from build123d import *

# Parameters (mm, degrees)
SKETCH1_W           = 53.32
SKETCH1_H           = 53.32
BOSS_EXTRUDE1_DEPTH = 5.08
SKETCH2_W           = 5.08
SKETCH2_H           = 5.08
CUT_EXTRUDE1_DEPTH  = 5.08
CUT_EXTRUDE2_DEPTH  = 5.08


with BuildPart() as part:
    # Sketch1 → Boss-Extrude1 (new body)
    with BuildSketch(Plane(origin=(0, 0, 0), x_dir=(1, 0, 0), z_dir=(0, 1, 0))):
        with Locations((4.159716312, -8.981205674)):
            Rectangle(SKETCH1_W, SKETCH1_H)
    extrude(amount=BOSS_EXTRUDE1_DEPTH)

    # Sketch2 → Cut-Extrude1 (cut)
    with BuildSketch(Plane(origin=(0, 5.08, 0), x_dir=(1, 0, 0), z_dir=(0, 1, 0))):
        with Locations((-13.620283688, -33.101205674)):
            Rectangle(SKETCH2_W, SKETCH2_H)
        with Locations((11.779716312, -33.101205674)):
            Rectangle(SKETCH2_W, SKETCH2_H)
        with Locations((21.939716312, -33.101205674)):
            Rectangle(SKETCH2_W, SKETCH2_H)
        with Locations((-3.460283688, -33.101205674)):
            Rectangle(SKETCH2_W, SKETCH2_H)
        with Locations((-19.960283688, 8.798794326)):
            Rectangle(SKETCH2_W, SKETCH2_H)
        with Locations((-19.960283688, -16.601205674)):
            Rectangle(SKETCH2_W, SKETCH2_H)
        with Locations((-19.960283688, -26.761205674)):
            Rectangle(SKETCH2_W, SKETCH2_H)
        with Locations((-19.960283688, -1.361205674)):
            Rectangle(SKETCH2_W, SKETCH2_H)
        with Locations((21.939716312, 15.138794326)):
            Rectangle(SKETCH2_W, SKETCH2_H)
        with Locations((-3.460283688, 15.138794326)):
            Rectangle(SKETCH2_W, SKETCH2_H)
        with Locations((-13.620283688, 15.138794326)):
            Rectangle(SKETCH2_W, SKETCH2_H)
        with Locations((11.779716312, 15.138794326)):
            Rectangle(SKETCH2_W, SKETCH2_H)
        with Locations((28.279716312, -26.761205674)):
            Rectangle(SKETCH2_W, SKETCH2_H)
        with Locations((28.279716312, -1.361205674)):
            Rectangle(SKETCH2_W, SKETCH2_H)
        with Locations((28.279716312, 8.798794326)):
            Rectangle(SKETCH2_W, SKETCH2_H)
        with Locations((28.279716312, -16.601205674)):
            Rectangle(SKETCH2_W, SKETCH2_H)
    extrude(amount=-CUT_EXTRUDE1_DEPTH, mode=Mode.SUBTRACT)

    # Sketch3 → Cut-Extrude2 (cut)
    with BuildSketch(Plane(origin=(0, 5.08, 0), x_dir=(1, 0, 0), z_dir=(0, 1, 0))):
        Polygon((4.159716312, -1.361205674), (6.699716312, -1.361205674), (6.699716312, -6.441205674), (11.779716312, -6.441205674), (11.779716312, -8.981205674), (11.779716312, -11.521205674), (6.699716312, -11.521205674), (6.699716312, -16.601205674), (4.159716312, -16.601205674), (1.619716312, -16.601205674), (1.619716312, -11.521205674), (-3.460283688, -11.521205674), (-3.460283688, -8.981205674), (-3.460283688, -6.441205674), (1.619716312, -6.441205674), (1.619716312, -1.361205674), align=None)
    extrude(amount=-CUT_EXTRUDE2_DEPTH, mode=Mode.SUBTRACT)


solid = part.part
Source: CAD feature listing. Evaluate the final solid. Frame: model axes, mm. A direction names the side the tool comes from. Give positions to 0.01 mm unless a question says otherwise; leave off trailing zeros. Write each loop counter-clockwise with the first axis right and the second up, starting at its lowest first coordinate (ties: lowest second). Pieces come first, ordered by that corner, then holes. Notation, with made-up numbers: (-24, 58.5) - (4, 58.5) arc R31 cw to (4, 97.5) - close; hole circle Ø4 at (70, 37.5). An arc over 180 degrees is marked (long way). Write item = value, one per line. Start each with the question number.
Q1. Material intervals for probe 1 along Z at (x, y) = (-18.5, 4.35); probe 2 along X at (y, z) = (0.3, -14); probe 3 along Z at (x, y) = (11, 4.65), sorted ascending.
Q2. Reachability of faces 4 (the flat face through (-14, 3, -12.599)), 5 (the flat face through (-6, 3, 33)), 6 (the flat face through (-20, 3, 3.901)), 7 (the flat face through (28, 3, -6.259)), 8 (the flat face through (9, 3, 6.441)) from +Z, -Z, +X, -X, +Y, -Y: full face, straight path, thin tool, end or side. Return the list, or none.
Q3. Pin query (flat end, axial travel): pin 1 Ø2.5 at (y, z) = (2.5, 26) entering from -X. Return the tip coordinate at first contact, or that it passes through.
Q4. Cut plane C-C, the plane x = 27. Return loops of the section in (y, z), then the cut area to 3 significant figures.
Q5. Cut plane A-A, the plane z = 5. Return loops of the section in (x, y), then the cut area to 3 significant figures.
Q6. Draft query along X for faces 1 (the flat face through (12, 3, -12.599)), 2 (the flat face through (30.82, 3, 33)), 3 (the flat face through (28, 3, -1.179)). Return one class per face: +X half, -X half, draft (parallel to the pull), parting line (faces both ways), or undercut.
Q7. Cut plane B-B, the plane x = 7.5. Return loops of the section in (y, z), then the cut area to 3 significant figures.
Computed values:
q1.probe_1 = -17.68 to -11.34, -6.26 to -1.18, 3.9 to 14.06, 19.14 to 24.22, 29.3 to 35.64
q1.probe_2 = -22.5 to -16.16, -11.08 to -6, -0.92 to 9.24, 14.32 to 19.4, 24.48 to 30.82
q1.probe_3 = -12.6 to 6.44, 11.52 to 30.56
q2.face_4 = -Z, +Y, -Y
q2.face_5 = +Z, +Y, -Y
q2.face_6 = -X, +Y, -Y
q2.face_7 = +X, +Y, -Y
q2.face_8 = +Y, -Y
q3.pin_1 = -17.42
q4.outline = (0, -17.68) - (5.08, -17.68) - (5.08, -11.34) - (0, -11.34) - close; (0, -6.26) - (5.08, -6.26) - (5.08, -1.18) - (0, -1.18) - close; (0, 3.9) - (5.08, 3.9) - (5.08, 14.06) - (0, 14.06) - close; (0, 19.14) - (5.08, 19.14) - (5.08, 24.22) - (0, 24.22) - close; (0, 29.3) - (5.08, 29.3) - (5.08, 35.64) - (0, 35.64) - close
q4.area = 168 mm²
q5.outline = (-22.5, 0) - (1.62, 0) - (1.62, 5.08) - (-22.5, 5.08) - close; (6.7, 0) - (30.82, 0) - (30.82, 5.08) - (6.7, 5.08) - close
q5.area = 245 mm²
q6.face_1 = undercut
q6.face_2 = +X half
q6.face_3 = draft
q7.outline = (0, -17.68) - (5.08, -17.68) - (5.08, 6.44) - (0, 6.44) - close; (0, 11.52) - (5.08, 11.52) - (5.08, 35.64) - (0, 35.64) - close
q7.area = 245 mm²
